Autodesk Inventor part; units mm, degrees
ref_plane "YZ Plane" through (0, 0, 0) normal (1, 0, 0) x (0, 1, 0)
ref_plane "XZ Plane" through (0, 0, 0) normal (0, 1, 0) x (-1, 0, 0)
ref_plane "XY Plane" through (0, 0, 0) normal (0, 0, 1) x (1, 0, 0)
sketch "Sketch1" plane through (0, 0, 0) normal (0, 0, 1) x (1, 0, 0)
  line L0 (0, 0) -> (25, 0)
  line L1 (25, 0) -> (25, 40)
  line L2 (25, 40) -> (0, 40)
  line L3 (0, 40) -> (0, 0)
  dimension "d1" = 25
  dimension "d2" = 40
  dimension "d3" = 25
extrude "Extrusion1" add sketch "Sketch1" against normal blind 30
sketch "Sketch2" plane through (25, 0, 0) normal (1, 0, 0) x (0, 0, -1)
  line L0 (0, 0) -> (30, 0)
  circle A0 centre (15, 6.56) radius 2.46
extrude "Extrusion2" cut sketch "Sketch2" against normal blind 30
sketch "Sketch3" plane through (0, 0, 0) normal (-1, 0, 0) x (0, 0, 1)
  line L0 (0, 0) -> (-30, 0)
  line L1 (-25.05, 0) -> (-4.95, 0)
  line L2 (-4.95, 0) -> (-4.95, 33.12)
  line L3 (-4.95, 33.12) -> (-25.05, 33.12)
  line L4 (-25.05, 33.12) -> (-25.05, 0)
  dimension "d11" = 20.1
extrude "Extrusion3" cut sketch "Sketch3" against normal blind 20
sketch "Sketch4" plane through (0, 0, 0) normal (0, -1, 0) x (1, 0, 0)
  line L0 (20, -4.95) -> (20, -25.05)
  line L1 (20, -15) -> (25, -15)
  line L2 (25, 0) -> (25, -30)
  line L3 (20, -8.025) -> (25, -8.025)
  line L4 (25, -8.025) -> (25, -21.975)
  line L5 (25, -21.975) -> (20, -21.975)
  line L6 (20, -21.975) -> (20, -8.025)
  line L7 (20, -8.025) -> (25, -21.975) construction
  line L8 (25, -8.025) -> (20, -21.975) construction
  line L9 (25, -12.54) -> (25, -17.46)
  point P0 (0, 0)
  point P1 (22.5, -15)
  dimension "d14" = 13.95
extrude "Extrusion4" add sketch "Sketch4" along normal blind 15
sketch "Sketch5" plane through (20, 0, 0) normal (-1, 0, 0) x (0, 0, 1)
  circle A0 centre (-15, 6.56) radius 2.46
  circle A1 centre (-15, 6.56) radius 4.7025
  circle A2 centre (-15, 6.56) radius 2.46
  circle A3 centre (-15, 6.56) radius 2.46
  point P0 (0, 0)
  dimension "d17" = 9.405
extrude "Extrusion5" cut sketch "Sketch5" against normal blind 2.1
sketch "Sketch6" plane through (25, 0, 0) normal (1, 0, 0) x (0, 0, -1)
  circle A0 centre (15, 6.56) radius 4.7025
  line L0 (15, 6.56) -> (15, 23.56)
  circle A1 centre (15, 23.56) radius 2.46
  point P0 (0, 0)
  dimension "d20" = 17
  dimension "d21" = 4.92
extrude "Extrusion6" cut sketch "Sketch6" against normal blind 10 contours A1
sketch "Sketch7" plane through (20, 0, 0) normal (-1, 0, 0) x (0, 0, 1)
  circle A0 centre (-15, 23.56) radius 2.46
  circle A1 centre (-15, 23.56) radius 4.7025
  point P0 (0, 0)
  dimension "d24" = 9.405
extrude "Extrusion7" cut sketch "Sketch7" against normal blind 2.1
sketch "Sketch9" plane through (25, 0, 0) normal (1, 0, 0) x (0, 0, -1)
  circle A0 centre (15, 6.56) radius 2.46
  circle A1 centre (15, 6.56) radius 2.46
  circle A2 centre (15, 23.56) radius 2.46
  circle A3 centre (15, 23.56) radius 2.46
  line L0 (30, 40) -> (30, 0)
  line L1 (30, 0) -> (30, 40)
  line L2 (30, 40) -> (0, 40)
  line L3 (0, 40) -> (0, 0)
  line L4 (0, 0) -> (8.025, 0)
  line L5 (21.975, 0) -> (21.975, -15)
  line L6 (21.975, -15) -> (8.025, -15)
  line L7 (8.025, -15) -> (8.025, 0)
  line L8 (0, 0) -> (8.025, 0)
  line L9 (21.975, 0) -> (30, 0)
extrude "Extrusion8" add sketch "Sketch9" along normal blind 5
sketch "Sketch10" plane through (0, 40, 0) normal (0, 1, 0) x (1, 0, 0)
  line L0 (0, 30) -> (30, 30)
  line L1 (30, 0) -> (0, 0)
  line L2 (0, 30) -> (30, 30)
  line L3 (30, 30) -> (30, 0)
  line L4 (30, 0) -> (0, 0)
  line L5 (0, 0) -> (0, 30)
extrude "Extrusion9" add sketch "Sketch10" along normal blind 30
sketch "Sketch12" plane through (30, 0, 0) normal (1, 0, 0) x (0, 0, -1)
  circle A0 centre (15, 6.56) radius 2.46
  line L0 (15, 6.56) -> (15, 15.06)
  circle A1 centre (15, 15.06) radius 2.525
  point P0 (0, 0)
  dimension "d31" = 8.5
  dimension "d33" = 5.05
extrude "Extrusion10" cut sketch "Sketch12" against normal blind 30 contours A1
sketch "Sketch14" plane through (0, 0, 0) normal (0, 0, 1) x (1, 0, 0)
  line L0 (30, 70) -> (0, 70)
  line L1 (0, 70) -> (0, 85)
  line L2 (-15, 100) -> (-23, 100)
  line L3 (30, 100) -> (15, 115)
  line L4 (-23, 115) -> (15, 115)
  line L5 (30, 0) -> (30, 70)
  line L6 (30, 100) -> (30, 70)
  line L7 (-20.5, 113.5) -> (-23, 115)
  line L8 (-20.5, 101.5) -> (-23, 100)
  line L9 (-18, 107.5) -> (-20.5, 101.5)
  line L10 (-18, 107.5) -> (-20.5, 113.5)
  arc A0 (0, 85) -> (-15, 100) centre (-15, 85) ccw
  point P0 (0, 0)
  point P1 (0, 100)
  dimension "d47" = 30
  dimension "d49" = 15
  dimension "d54" = 15
extrude "Extrusion12" add sketch "Sketch14" against normal blind 30
sketch "Sketch15" plane through (0, 0, -25.05) normal (-1, 0, 0) x (0, 0, 1)
  line L0 (0, 33.12) -> (20.1, 33.12)
  line L1 (20.1, 33.12) -> (20.1, 0)
  line L2 (0, 33.12) -> (20.1, 33.12)
  line L3 (20.1, 33.12) -> (20.1, 31.1)
  line L4 (20.1, 31.1) -> (0, 31.1)
  line L5 (0, 31.1) -> (0, 33.12)
  point P0 (25.05, 0)
  dimension "d57" = 2.02
extrude "Extrusion13" add sketch "Sketch15" against normal blind 20
properties part number "10mm_x_30mm"
For this review, take the finished solid that the model builds, in its own axes (mm). A direction names the side the tool comes from. Round coordinates to 2 decimals unless told otherwise and drop trailing zeros. Write each loop counter-clockwise with the first axis right and the second up, starting at its lowest first coordinate (ties: lowest second). Pieces come first, ordered by that corner, then holes.
1) Mouldability with a two-part tool opening along Y and no side actions: class faces 1 (the face through (23, 107, -15)), 2 (the face through (25.07, 15.171, -12.477)), 3 (the face through (25, -15, -15)), 4 (the face through (25.995, 24.502, -17.272)) as +Y half, -Y half, draft (parallel to the pull), parting line (faces both ways), or undercut.
Answer below:
face 1: +Y half
face 2: undercut
face 3: -Y half
face 4: undercut
2) Take a section at D-D on x = -13. Give the boundary of the cut face in (y, z), then the cut area to 3 significant figures.
Answer below:
outline: (99.87, -30) - (115, -30) - (115, 0) - (99.87, 0) - close
area: 454 mm2
3) For line 1 along Y through (x, z) = (28.5, -15) (3 decimals); line 2 along Y through (x, z) = (27.5, -14); line 3 along Z through (x, y) = (24, 15.06) (3 decimals), list the stretches that pass through material, from the lowest coordinate up.
Answer below:
line 1: y = -15 to 4.1, 9.02 to 12.535, 17.585 to 21.1, 26.02 to 101.5
line 2: y = -15 to 4.31, 8.81 to 12.74, 17.38 to 21.31, 25.81 to 102.5
line 3: z = -30 to -17.525, -12.475 to 0
4) Take a section at C-C on y = 51.5. Give the boundary of the cut face in (x, z), then the cut area to 3 significant figures.
Answer below:
outline: (0, -30) - (30, -30) - (30, 0) - (0, 0) - close
area: 900 mm2
5) Machinability: for faces 5 (the face through (25, -7, -21.975)), 6 (the face through (20, 8, -20)), 7 (the face through (21.035, 27.525, -12.472)), 8 (the face through (25, -8, -8.025)), which of the approach directions +Z, -Z, +X, -X, +Y, -Y give a long, thin tool a straight path to every point of the face, cutting with its end or side? Answer none if there is none.
Answer below:
face 5: -Z, +X, -X, -Y
face 6: -X, -Y
face 7: -X
face 8: +Z, +X, -X, -Y
6) Take a section at A-A on y = 23.56. Give the boundary of the cut face in (x, z), then the cut area to 3 significant figures.
Answer below:
outline: (0, -30) - (30, -30) - (30, -17.46) - (22.1, -17.46) - (22.1, -19.7) - (20, -19.7) - (20, -25.05) - (0, -25.05) - close; (0, -4.95) - (20, -4.95) - (20, -10.3) - (22.1, -10.3) - (22.1, -12.54) - (30, -12.54) - (30, 0) - (0, 0) - close
area: 439 mm2
7) Take a section at B-B on x = 5. Give the boundary of the cut face in (y, z).
Answer below:
outline: (0, -30) - (115, -30) - (115, 0) - (0, 0) - (0, -4.95) - (31.1, -4.95) - (31.1, -25.05) - (0, -25.05) - close
8) Insertion check: pin 1 Ø5.5 at (y, z) = (6.56, -15) entering from -X; pin 2 Ø11 at (x, y) = (25.5, -10.5) entering from +Z (3 decimals); pin 3 Ø2.5 at (x, z) = (14, -27.5) entering from -Y. Each pin has a flat end and moves straight along its axis. Give the tip position at first contact, or say it passes through.
Answer below:
pin 1: stops at x = 22.1
pin 2: stops at z = -8.025
pin 3: stops at y = 0
